Source: three-view drawing plus pictorial views. Frame: mm from the lowest corner of the part. A direction names the side the tool comes from. Give positions to 0.01 mm unless a question says otherwise; leave off trailing zeros. Order: outer loops, then holes, each group sorted by start corner. A loop starts at its lowest first (then second) coordinate and runs counter-clockwise, first axis right, second up. Notation, with made-up numbers: M 80,21.25 L 130,21.25 A19 ccw 130,51.25 Z; hole C 18,1 d4. An arc over 180 degrees is marked long. One line per item, written item: value. Start each with the question number.
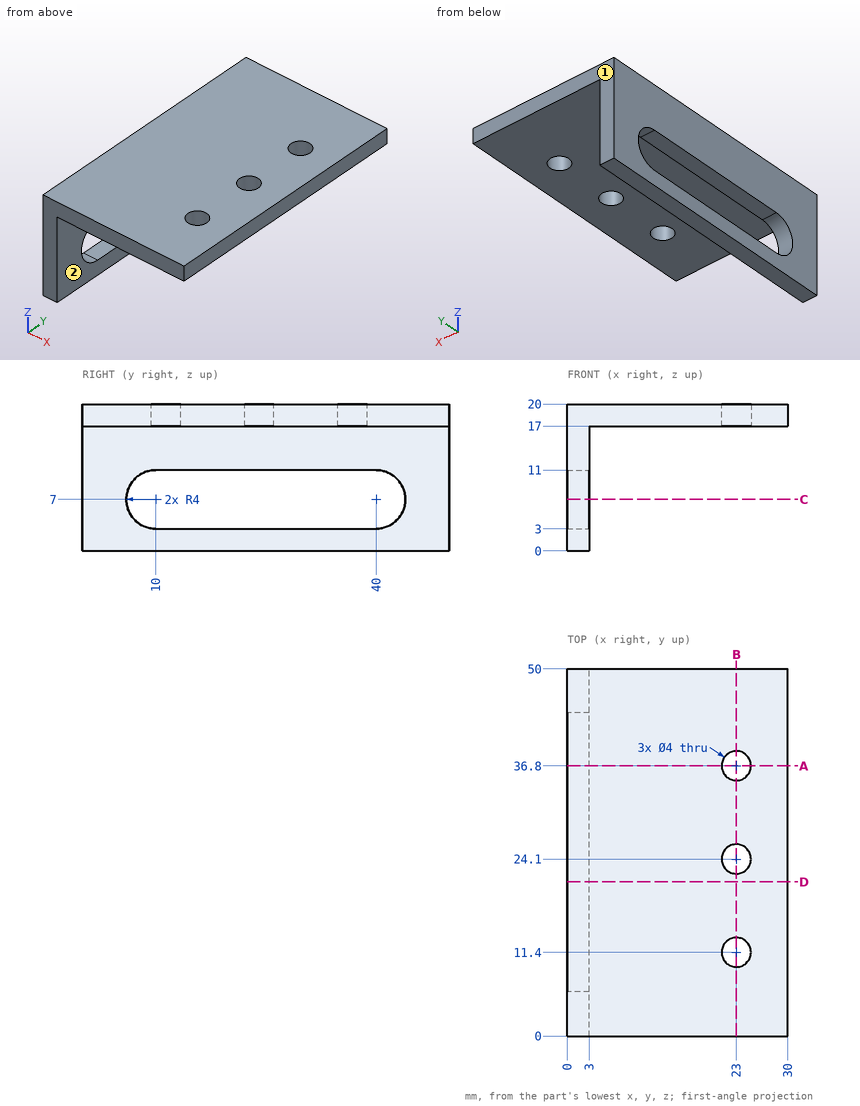
Q1. Section query D-D on y = 21. Return loops of the section in (x, z).
Q2. Contact query for flat-ended pins moving along their axis: pin 1 (12 mm diameter, centred on x = 19.5, z = 8, fed in from -Y); pin 2 (8 mm diameter, centred on x = 23.5, y = 36.5, fed in from -Z); pin 3 (8.5 mm diameter, centred on y = 12.5, z = 5.5, fed in from +X). Output: stop coordinate, or through.
Q3. Ray query, line 1 along Y through (x, z) = (23, 17.75); line 2 along Y through (x, z) = (22.25, 18.5); line 3 along Z through (x, y) = (24.5, 16). Return the intervals inside material, ascending. Write a range as [from, to].
Q4. Section query C-C on z = 7. Return loops of the section in (x, y).
Q5. Section query B-B on x = 23. Return loops of the section in (y, z).
Q6. Set-up query: the marked faces 1 and 2. Return all of +Z, -Z, +X, -X, +Y, -Y with unobstructed straight access to the full face (end or side cutting, diameter ignored); none if empty.
Q7. Section query A-A on y = 36.8. Return loops of the section in (x, z), and give its area (3 significant figures).
Results below:
1. outline: M 0,0 L 3,0 L 3,3 L 0,3 Z; M 0,11 L 3,11 L 3,17 L 30,17 L 30,20 L 0,20 Z
2. pin 1: through
2. pin 2: z = 17
2. pin 3: x = 3
3. line 1: [0, 9.4], [13.4, 22.1], [26.1, 34.8], [38.8, 50]
3. line 2: [0, 9.55], [13.25, 22.25], [25.95, 34.95], [38.65, 50]
3. line 3: [17, 20]
4. outline: M 0,0 L 3,0 L 3,6 L 0,6 Z; M 0,44 L 3,44 L 3,50 L 0,50 Z
5. outline: M 0,17 L 9.4,17 L 9.4,20 L 0,20 Z; M 13.4,17 L 22.1,17 L 22.1,20 L 13.4,20 Z; M 26.1,17 L 34.8,17 L 34.8,20 L 26.1,20 Z; M 38.8,17 L 50,17 L 50,20 L 38.8,20 Z
6. face 1: +Z, -Z, +X, -X, +Y
6. face 2: -Z, +X, +Y, -Y
7. outline: M 0,0 L 3,0 L 3,3 L 0,3 Z; M 0,11 L 3,11 L 3,17 L 21,17 L 21,20 L 0,20 Z; M 25,17 L 30,17 L 30,20 L 25,20 Z
7. area: 105 mm2
